Here's how the part is built. I have some questions about the finished solid (model axes, mm). Face numbers are marked on the shaded views. Give positions to 0.01 mm unless a question says otherwise; leave off trailing zeros. Loops run counter-clockwise (first coordinate to the right, second up) from the corner with the lowest first, then second, coordinate; pieces in that order, holes last.
Q1. If we section it at C-C (y = 11.5): Please give me the cut outline in (x, z).
Q2. If we section it at B-B (x = 0): Please give me the cut outline in (y, z).
Q3. If we section it at A-A (z = 0): Please give me the cut outline in (x, y), plus the area to 3 significant figures.
Q4. We'd pull the mould along Z, two halves only. Please class the marked faces 1, 2 and 3: +Z half, -Z half, draft (parallel to the pull), parting line (faces both ways), or undercut.
Q5. Will these pins go through, and if not, where does the flat tip stop? P1, Ø5, axis at y = -2.5, z = 6.5, coming from the -X side; P2, Ø10, axis at y = -5, z = -4, coming from the -X side; P3, Ø6, axis at y = 0.89, z = 0, coming from the -X side; P4, Ø8, axis at y = 10, z = -5, coming from the +X side.
Q6. If we section it at D-D (y = 2.75): Please give me the cut outline in (x, z), plus the area to 3 significant figures.
Q7. I need wall thicknesses on line 1 (Z direction, x = 0.5, y = -2.5); line 2 (Y direction, x = -10.5, z = 4); line 3 (Z direction, x = 3, y = 9). Which ranges of each line are inside material? Lowest first, please.
from build123d import *

# Parameters (mm, degrees)
F0_R      = 15.940718
F1_DEPTH  = 12
F1_FACE_R = 15.940718
F2_DEPTH  = 15
F3_R      = 14.322949
F4_DEPTH  = 25
F5_R      = 5
F6_R      = 4.914735
F7_DEPTH  = 15.941718


with BuildPart() as f1:
    # F0 (on Front) → F1 (new body)
    with BuildSketch(Plane.XZ):
        Circle(F0_R)
    extrude(amount=F1_DEPTH)

    # F1_face (on face) → F2 (join)
    with BuildSketch(Plane(origin=(0, 0, 0), x_dir=(1, 0, 0), z_dir=(0, 1, 0))):
        Circle(F1_FACE_R)
    extrude(amount=F2_DEPTH)

    # F3 (on face) → F4 (cut)
    with BuildSketch(Plane(origin=(0, 15, 0), x_dir=(-1, 0, 0), z_dir=(0, 1, 0))):
        Circle(F3_R)
    extrude(amount=-F4_DEPTH, mode=Mode.SUBTRACT)

    # F5
    f5_edges = [f1.edges().sort_by_distance(p)[0] for p in [
        (-15.940718, -12, 0),
    ]]
    fillet(f5_edges, radius=F5_R)

    # F6 (on Right) → F7 (cut, through all)
    with BuildSketch(Plane.YZ):
        with Locations((0.894999, 0)):
            Circle(F6_R)
    extrude(amount=-F7_DEPTH, mode=Mode.SUBTRACT)


solid = f1.part
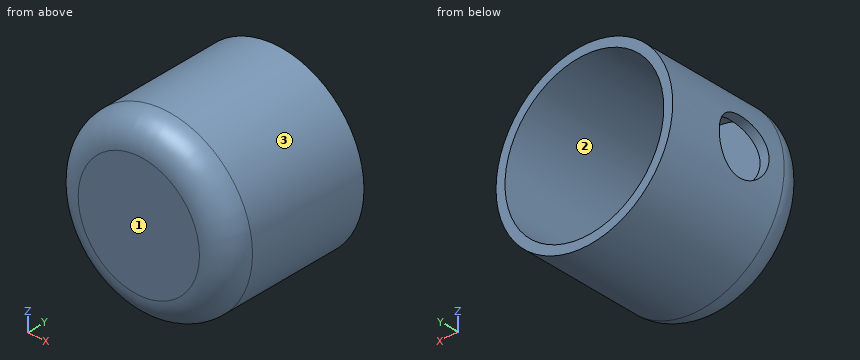
Check sheet entries:
1. outline: circle Ø31.88 at (0, 0); hole circle Ø28.65 at (0, 0)
2. outline: (-12, -10.94) arc R5 ccw to (-7, -15.94) - (15, -15.94) - (15, -14.32) - (-10, -14.32) - (-10, 14.32) - (15, 14.32) - (15, 15.94) - (-7, 15.94) arc R5 ccw to (-12, 10.94) - close
3. outline: (-15.94, -7) arc R5 ccw to (-10.94, -12) - (10.94, -12) arc R5 ccw to (15.94, -7) - (15.94, 15) - (14.32, 15) - (14.32, -10) - (-14.32, -10) - (-14.32, -4.02) - (-15.94, -4.02) - close; (-15.94, 5.81) - (-14.32, 5.81) - (-14.32, 15) - (-15.94, 15) - close
3. area: 118 mm2
4. face 1: draft
4. face 2: undercut
4. face 3: parting line
5. P1: stops at x = -15.43
5. P2: stops at x = -15.94
5. P3: stops at x = 14.01
5. P4: stops at x = 15.91
6. outline: (-15.28, -4.55) arc R15.94 ccw (long way) to (-15.28, 4.55) - (-13.58, 4.55) arc R14.32 cw (long way) to (-13.58, -4.55) - close
6. area: 139 mm2
7. line 1: z = -15.93 to -14.31, 14.31 to 15.93
7. line 2: y = -11.99 to -10
7. line 3: z = -15.66 to -14.01, 14.01 to 15.66
